Source: CAD feature listing. Evaluate the final solid. Frame: model axes, mm. A direction names the side the tool comes from. Coordinates: 2 decimals unless noted, no trailing zeros. Write each loop counter-clockwise with the first axis right and the second up, starting at its lowest first coordinate (ties: lowest second). Pieces come first, ordered by that corner, then holes. Notation, with made-up numbers: M 77,5.25 L 90,5.25 A28 ccw 90,44.25 Z; hole C 68.5,33.5 d1. An arc over 180 degrees is marked long. Write item = value, one per line. Start each with the question number.
1. Pull-direction query (Y, two-part tool) for faces 4 (the face through (-70, 0, 6)), 5 (the face through (170, -1, 6)), 6 (the face through (-2, 57.5, 6)); classes: pulls with the +Y half, pulls with the -Y half, needs draft (parallel to the pull), parting line crosses it, or undercut.
2. Section query B-B (y = 37.5). Output: boundary loops of the cut face in (x, z), then the cut area to 3 significant figures.
3. Section query D-D (y = 3.5). Output: boundary loops of the cut face in (x, z), then the cut area to 3 significant figures.
4. Section query A-A (x = 142.5). Output: boundary loops of the cut face in (y, z), then the cut area to 3 significant figures.
5. Line query: line 1 along Y through (x, z) = (-142.5, 1.6); line 2 along Y through (x, z) = (15, 8.5); line 3 along X through (y, z) = (38.5, 7.5). Output: solid intervals per line, ascending.
6. Pin query (flat end, axial travel): pin 1 Ø7 at (x, y) = (-142, 40) entering from +Z; pin 2 Ø7 at (x, y) = (142.5, -22.5) entering from +Z. Return the tip coordinate at first contact, or that it passes through.
7. Access query for faces 1 (the face through (147, 36, 3)), 2 (the face through (-2, 26, 12)), 3 (the face through (66.99, 22.15, 6.08)). Directions: +Z, -Z, +X, -X, +Y, -Y. A direction counts if a zero-diameter tool reaches every point of the face in a straight line with its end or side. Return the directions, or none.
8. Section query C-C (z = 7). Output: boundary loops of the cut face in (x, y).
```python
from build123d import *

# Parameters (mm, degrees)
SKETCH_1_W                = 340
SKETCH_1_H                = 115
EXTRUDE_1_DEPTH           = 12
HOLE_WIZARD_1_D           = 9
HOLE_WIZARD_1_CBORE_D     = 14
HOLE_WIZARD_1_CBORE_DEPTH = 9
CUT_EXTRUDE_1_DEPTH       = 13


with BuildPart() as part:
    # 草图1 → 凸台-拉伸1 (new body)
    with BuildSketch(Plane.XY):
        Rectangle(SKETCH_1_W, SKETCH_1_H)
    extrude(amount=EXTRUDE_1_DEPTH)

    # 打孔尺寸(%根据)内六角圆柱头螺钉的类型1 (through all)
    with Locations(Plane.XY.offset(12)):
        with Locations((-142.5, 37.5), (142.5, 37.5), (142.5, -22.5), (-142.5, -22.5)):
            CounterBoreHole(HOLE_WIZARD_1_D / 2, HOLE_WIZARD_1_CBORE_D / 2, HOLE_WIZARD_1_CBORE_DEPTH)

    # 草图4 → 切除-拉伸1 (cut, through all)
    with BuildSketch(Plane.XY.offset(12)):
        with BuildLine():
            Line((-60, 25), (60, 25))
            ThreePointArc((60, 25), (67.071067812, 22.071067812), (70, 15))
            Line((70, 15), (70, -15))
            ThreePointArc((70, -15), (67.071067812, -22.071067812), (60, -25))
            Line((60, -25), (-60, -25))
            ThreePointArc((-60, -25), (-67.071067812, -22.071067812), (-70, -15))
            Line((-70, -15), (-70, 15))
            ThreePointArc((-70, 15), (-67.071067812, 22.071067812), (-60, 25))
        make_face()
    extrude(amount=-CUT_EXTRUDE_1_DEPTH, mode=Mode.SUBTRACT)


solid = part.part
```
Results are:
q1.face_4 = undercut
q1.face_5 = needs draft
q1.face_6 = pulls with the +Y half
q2.outline = M -170,0 L -147,0 L -147,3 L -149.5,3 L -149.5,12 L -170,12 Z; M -138,0 L 138,0 L 138,3 L 135.5,3 L 135.5,12 L -135.5,12 L -135.5,3 L -138,3 Z; M 147,0 L 170,0 L 170,12 L 149.5,12 L 149.5,3 L 147,3 Z
q2.area = 3,770 mm^2
q3.outline = M -170,0 L -70,0 L -70,12 L -170,12 Z; M 70,0 L 170,0 L 170,12 L 70,12 Z
q3.area = 2,400 mm^2
q4.outline = M -57.5,0 L -27,0 L -27,3 L -29.5,3 L -29.5,12 L -57.5,12 Z; M -18,0 L 33,0 L 33,3 L 30.5,3 L 30.5,12 L -15.5,12 L -15.5,3 L -18,3 Z; M 42,0 L 57.5,0 L 57.5,12 L 44.5,12 L 44.5,3 L 42,3 Z
q4.area = 1,070 mm^2
q5.line_1 = -57.5 to -27, -18 to 33, 42 to 57.5
q5.line_2 = -57.5 to -25, 25 to 57.5
q5.line_3 = -170 to -149.43, -135.57 to 135.57, 149.43 to 170
q6.pin_1 = 3
q6.pin_2 = through
q7.face_1 = +Z
q7.face_2 = +Z, +X, -X, +Y, -Y
q7.face_3 = +Z, -Z
q8.outline = M -170,-57.5 L 170,-57.5 L 170,57.5 L -170,57.5 Z; hole C -142.5,-22.5 d14; hole C -142.5,37.5 d14; hole M -70,-15 A10 ccw -60,-25 L 60,-25 A10 ccw 70,-15 L 70,15 A10 ccw 60,25 L -60,25 A10 ccw -70,15 Z; hole C 142.5,-22.5 d14; hole C 142.5,37.5 d14
